The drawing under review shows one solid part. Ordinate dimensions are in mm from its lowest x, y, z. A direction names the side the tool comes from. Round coordinates to 2 decimals unless told otherwise and drop trailing zeros. Order: outer loops, then holes, each group sorted by start corner. A loop starts at its lowest first (then second) coordinate and runs counter-clockwise, first axis right, second up. Notation, with made-up numbers: (30, -33.5) - (83, -33.5) arc R33 cw to (83, -1.5) - close; hole circle Ø7 at (14.25, 37). An arc over 180 degrees is marked (long way). One line per question, with ' | ' between items.
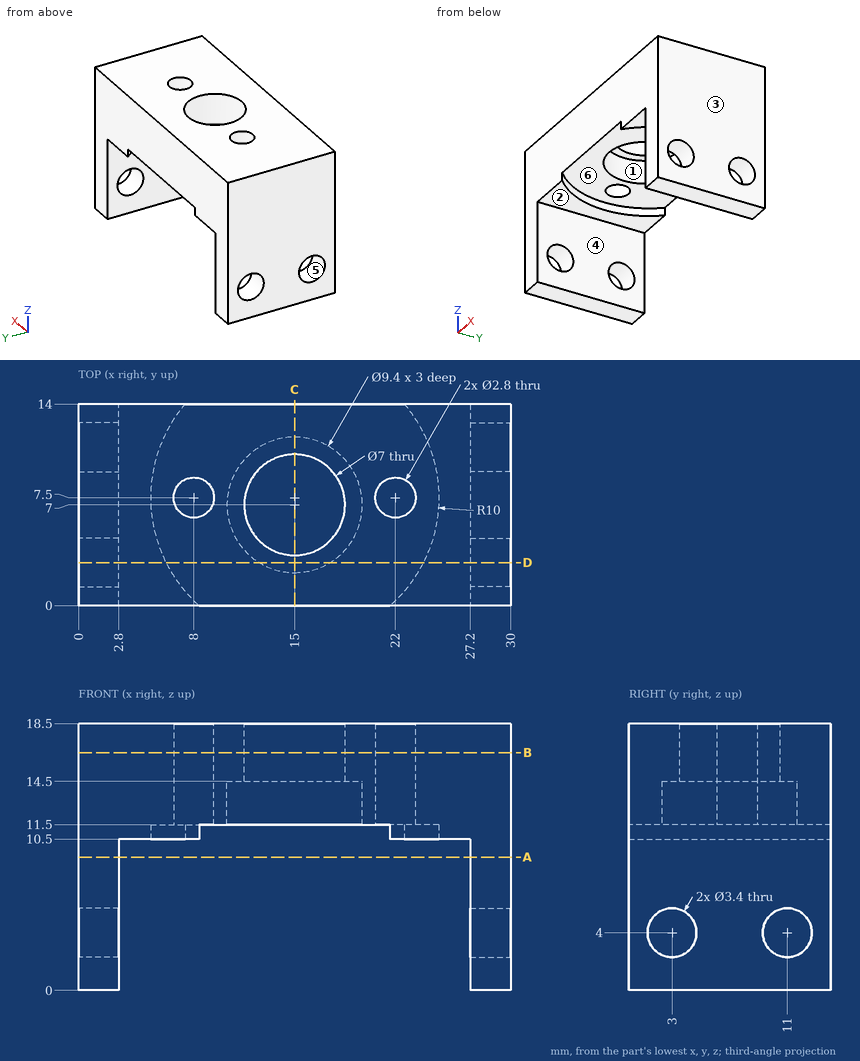
(1) We need section D-D on y = 3. State the section outline as (x, z) points, plus the area to 3 significant figures.
Output values:
outline: (0, 0) - (2.8, 0) - (2.8, 2.3) - (0, 2.3) - close; (0, 5.7) - (2.8, 5.7) - (2.8, 10.5) - (6.07, 10.5) - (6.07, 11.5) - (12.53, 11.5) - (12.53, 14.5) - (17.47, 14.5) - (17.47, 11.5) - (23.93, 11.5) - (23.93, 10.5) - (27.2, 10.5) - (27.2, 5.7) - (30, 5.7) - (30, 18.5) - (0, 18.5) - close; (27.2, 0) - (30, 0) - (30, 2.3) - (27.2, 2.3) - close | area: 247 mm^2
(2) Mouldability with a two-part tool opening along Z and no side actions: class the marked faces 4, 5 and 6 as released by +Z, released by -Z, zero draft, split by the parting line, or undercut.
Output values:
face 4: zero draft | face 5: undercut | face 6: released by -Z
(3) We need section B-B on z = 16.5. State the section outline as (x, y) points, plus the area to 3 significant figures.
Output values:
outline: (0, 0) - (30, 0) - (30, 14) - (0, 14) - close; hole circle Ø2.8 at (8, 7.5); hole circle Ø7 at (15, 7); hole circle Ø2.8 at (22, 7.5) | area: 369 mm^2
(4) We need section C-C on x = 15. State the section outline as (y, z) points, plus the area to 3 significant figures.
Output values:
outline: (0, 11.5) - (2.3, 11.5) - (2.3, 14.5) - (3.5, 14.5) - (3.5, 18.5) - (0, 18.5) - close; (10.5, 14.5) - (11.7, 14.5) - (11.7, 11.5) - (14, 11.5) - (14, 18.5) - (10.5, 18.5) - close | area: 41.8 mm^2
(5) For the marked faces 1, 2 and 3, list the 3-axis set-ups (+Z, -Z, +X, -X, +Y, -Y) from which the entire face can be reached by the end or side of a thin tool; tool diameter is ignored.
Output values:
face 1: -Z | face 2: -Z, +Y, -Y | face 3: +Z, -Z, +X, +Y, -Y
(6) For probe 1 along Y at (x, z) = (27.9, 4); probe 2 along Z at (x, y) = (0.95, 3); probe 3 along Y at (x, z) = (15, 12.95), list the stretches that pass through material, from the lowest coordinate up. Write a range as [from, to].
Output values:
probe 1: [0, 1.3], [4.7, 9.3], [12.7, 14] | probe 2: [0, 2.3], [5.7, 18.5] | probe 3: [0, 2.3], [11.7, 14]
(7) We need section A-A on z = 9.25. State the section outline as (x, y) points.
Output values:
outline: (0, 0) - (2.8, 0) - (2.8, 14) - (0, 14) - close; (27.2, 0) - (30, 0) - (30, 14) - (27.2, 14) - close
(8) Insertion check: pin 1 (6 mm diameter, centred on x = 12.5, y = 8, fed in from +Z); pin 2 (3 mm diameter, centred on x = 8, y = 7.5, fed in from -Z); pin 3 (3 mm diameter, centred on x = 4.5, y = 6.5, fed in from -Z); pin 4 (4 mm diameter, centred on x = 14, y = 5, fed in from -Z). Each pin has a flat end and moves straight along its axis. Give the tip position at first contact, or say it passes through.
Output values:
pin 1: z = 18.5 | pin 2: z = 11.5 | pin 3: z = 10.5 | pin 4: z = 14.5
